Can you work these out from the model? Positions are in its coordinate system, mm. Face numbers are marked on the shaded views. Give positions to 0.01 mm unless a question says otherwise; leave off trailing zeros. Order: outer loops, then holes, each group sorted by start corner. A loop starts at its lowest first (then second) coordinate and runs counter-clockwise, first axis right, second up. Notation, with made-up numbers: (73.5, 31.25) - (94.5, 31.25) arc R10 cw to (94.5, 43.25) - close; hole circle Ø10 at (-8.75, 14.5). An arc over 180 degrees is marked (long way). Return JSON: item names as keys, results as strings.
```python
from build123d import *

# Parameters (mm, degrees)
ESQUISSE1_R             = 4
BOSS_EXTRU_1_DEPTH      = 2
CONG_1_R                = 1
ESQUISSE2_W             = 0.2
ESQUISSE2_H             = 3
BOSS_EXTRU_2_DEPTH      = 3.2
BOSS_EXTRU_3_DEPTH      = 10
BOSS_EXTRU_3_DEPTH_BACK = 10
ESQUISSE3_W             = 3
ESQUISSE3_H             = 0.2
CONG_2_R                = 1.5


with BuildPart() as part:
    # Esquisse1 → Boss.-Extru.1 (new body)
    with BuildSketch(Plane(origin=(0, 0, 0), x_dir=(1, 0, 0), z_dir=(0, 1, 0))):
        with Locations(Location((0, 0, 0), (0, 0, 270))):
            Circle(ESQUISSE1_R)
    extrude(amount=BOSS_EXTRU_1_DEPTH)

    # Congé1
    cong_1_edges = [part.edges().sort_by_distance(p)[0] for p in [
        (0, 2, -4),
    ]]
    fillet(cong_1_edges, radius=CONG_1_R)

    # Esquisse2 → Boss.-Extru.2 (add)
    with BuildSketch(Plane.XZ):
        with Locations((-0.3, 0)):
            Rectangle(ESQUISSE2_W, ESQUISSE2_H)
        with Locations((0.3, 0.05)):
            Rectangle(ESQUISSE2_W, ESQUISSE2_H)
    extrude(amount=BOSS_EXTRU_2_DEPTH)

    # Esquisse3 → Boss.-Extru.3 (add, two sides: drawn at the far end of the back side and taken through both)
    with BuildSketch(Plane.ZY.offset(0.4).offset(-BOSS_EXTRU_3_DEPTH_BACK)):
        with Locations((0, -3.1)):
            Rectangle(ESQUISSE3_W, ESQUISSE3_H)
    extrude(amount=BOSS_EXTRU_3_DEPTH + BOSS_EXTRU_3_DEPTH_BACK)

    # Congé2
    cong_2_edges = [part.edges().sort_by_distance(p)[0] for p in [
        (9.6, -3.1, -1.5),
        (9.6, -3.1, 1.5),
        (-10.4, -3.1, 1.5),
        (-10.4, -3.1, -1.5),
    ]]
    fillet(cong_2_edges, radius=CONG_2_R - 0.0001)  # a hair under: the kernel refuses the full size


solid = part.part
```
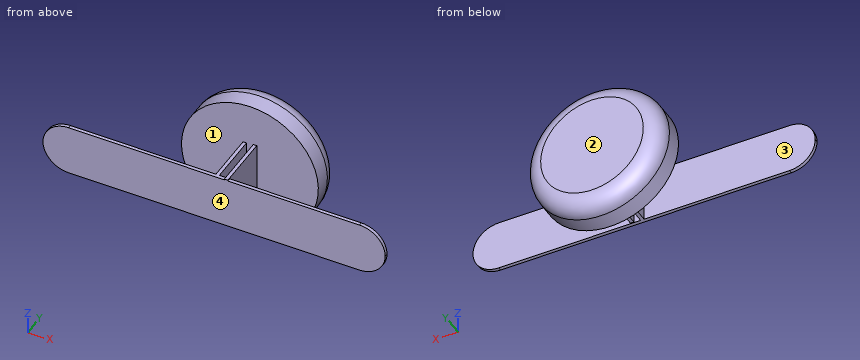
1. Suppose I cut it at B-B (y = 0.5). List the corners of the cut face in (x, z) for me.
Checks:
{"outline": "circle Ø8 at (0, 0)"}
2. Suppose I cut it at D-D (y = 1.75). List the corners of the cut face in (x, z) for me, plus the area to 3 significant figures.
Checks:
{"outline": "circle Ø7.32 at (0, 0)", "area": "42.1 mm^2"}
3. Thinking about a two-plate mould opening in Y: for the marked faces 1, 2, 3 and 4, which applies, +Y half, -Y half, draft (parallel to the pull), parting line (faces both ways), or undercut?
Checks:
{"face 1": "undercut", "face 2": "+Y half", "face 3": "undercut", "face 4": "-Y half"}
4. For pin 1 Ø1 at (x, y) = (-2, -2) entering from +Z (3 decimals); pin 2 Ø3 at (x, y) = (-2.5, 0.5) entering from +Z; pin 3 Ø1.5 at (y, z) = (-2, 2) entering from -X; pin 4 Ø1 at (y, z) = (0.5, 1.5) entering from +X, each with a flat end and sliding along its axis, tell me the tip position at first contact or that it passes through.
Checks:
{"pin 1": "through", "pin 2": "z = 3.87", "pin 3": "x = -0.4", "pin 4": "x = 3.87"}
5. Suppose I cut it at C-C (x = -6). List the corners of the cut face in (y, z) for me, plus the area to 3 significant figures.
Checks:
{"outline": "(-3.2, -1.5) - (-3, -1.5) - (-3, 1.5) - (-3.2, 1.5) - close", "area": "0.600 mm^2"}
6. Suppose I cut it at A-A (x = 0). List the corners of the cut face in (y, z) for me.
Checks:
{"outline": "(-3.2, -1.5) - (-3, -1.5) - (-3, 1.5) - (-3.2, 1.5) - close; (0, -4) - (1, -4) arc R1 ccw to (2, -3) - (2, 3) arc R1 ccw to (1, 4) - (0, 4) - close"}
7. If I drill on L1, parallel to X at y = -1.2, z = 0.25; L2, parallel to Y at x = 1.75, z = -1.25; L3, parallel to Z at x = 0.25, y = -2.1, over which ranges is the centre line in solid material (lowest first)? Write a range as [from, to].
Checks:
{"L1": "[-0.4, -0.2], [0.2, 0.4]", "L2": "[-3.2, -3], [0, 2]", "L3": "[-1.45, 1.55]"}
